```python
from build123d import *

# Parameters (mm, degrees)
SKETCH1_W           = 20
SKETCH1_H           = 25
BOSS_EXTRUDE1_DEPTH = 30
SKETCH2_W           = 40
SKETCH2_H           = 40
BOSS_EXTRUDE2_DEPTH = 20
FILLET1_R           = 10


with BuildPart() as part:
    # Sketch1 → Boss-Extrude1 (new body)
    with BuildSketch(Plane.XY):
        with Locations((-20, -12.5)):
            Rectangle(SKETCH1_W, SKETCH1_H)
    extrude(amount=BOSS_EXTRUDE1_DEPTH)

    # Sketch2 → Boss-Extrude2 (add)
    with BuildSketch(Plane.XY):
        with Locations((-10, -5)):
            Rectangle(SKETCH2_W, SKETCH2_H)
    extrude(amount=-BOSS_EXTRUDE2_DEPTH)

    # Fillet1
    fillet1_edges = [part.edges().sort_by_distance(p)[0] for p in [
        (-20, 0, 0),
    ]]
    fillet(fillet1_edges, radius=FILLET1_R)
    fillet1_2_edges = [part.edges().sort_by_distance(p)[0] for p in [
        (10, 15, -10),
        (-20, 0, 30),
    ]]
    fillet(fillet1_2_edges, radius=FILLET1_R)


solid = part.part
```
Could you check a few things on this model? Use its own coordinates, in mm. A direction names the side the tool comes from. Round coordinates to 2 decimals unless told otherwise and drop trailing zeros. Loops run counter-clockwise (first coordinate to the right, second up) from the corner with the lowest first, then second, coordinate; pieces in that order, holes last.
Q1. For P1, Ø8, axis at x = -24.5, z = 16.5, coming from the +Y side; P2, Ø3, axis at x = -4.5, y = -14.5, coming from the +Z side; P3, Ø24, axis at y = -3, z = 15, coming from the +X side, each with a flat end and sliding along its axis, tell me the tip position at first contact or that it passes through.
Q2. I want a section at A-A (x = -13.5). Write out the boundary of the cut face in (y, z).
Q3. I want a section at B-B (y = -12.5). Write out the boundary of the cut face in (x, z), and give its area (3 significant figures).
Q4. I want a section at C-C (z = 11.5). Write out the boundary of the cut face in (x, y).
Q5. Please list where these lines run through material, in increasing order: L1, parallel to X at y = -17.5, z = 7.5; L2, parallel to Z at x = 7.5, y = 9; L3, parallel to Y at x = -17.5, z = 19.5.
Q6. On a 3-axis mill with a long thin cutter (end or side, diameter ignored), from which of +Z, -Z, +X, -X, +Y, -Y can I reach the whole of each face in a straight line? I mean faces 1 (the flat face through (-10, -5, -20)), 2 (the flat face through (-10, -12, 15)), 3 (the flat face through (-20, 0, 15)), 4 (the flat face through (-1, -5, 0)), 5 (the flat face through (-15, 15, -10)). Say none if no direction works.
Q7. I want a section at D-D (y = -4). Write out the boundary of the cut face in (x, z), and give its area (3 significant figures).
Answer below:
1. P1: stops at y = 0
1. P2: stops at z = 0
1. P3: stops at x = -10
2. outline: (-25, -20) - (15, -20) - (15, 0) - (10, 0) arc R10 cw to (0, 10) - (0, 20) arc R10 ccw to (-10, 30) - (-25, 30) - close
3. outline: (-30, -20) - (10, -20) - (10, 0) - (-10, 0) - (-10, 30) - (-30, 30) - close
3. area: 1,400 mm2
4. outline: (-30, -25) - (-10, -25) - (-10, 0) - (-30, 0) - close
5. L1: x = -30 to -10
5. L2: z = -20 to 0
5. L3: y = -25 to 0
6. face 1: -Z, +X, -X, +Y, -Y
6. face 2: +Z, +X, +Y, -Y
6. face 3: +Z, +X, -X, +Y
6. face 4: +Z, +X, +Y
6. face 5: +Z, -Z, +X, -X, +Y
7. outline: (-30, -20) - (10, -20) - (10, 0) - (-10, 0) - (-10, 28) - (-30, 28) - close
7. area: 1,360 mm2
